Autodesk Inventor part; units mm, degrees
ref_plane "YZ Plane" through (0, 0, 0) normal (1, 0, 0) x (0, 1, 0)
ref_plane "XZ Plane" through (0, 0, 0) normal (0, 1, 0) x (-1, 0, 0)
ref_plane "XY Plane" through (0, 0, 0) normal (0, 0, 1) x (1, 0, 0)
sketch "Boceto1" plane through (0, 0, 0) normal (0, 1, 0) x (-1, 0, 0)
  line L0 (100, 80) -> (-100, 80)
  line L1 (-100, 80) -> (-100, -80)
  line L2 (-100, -80) -> (100, -80)
  line L3 (100, -80) -> (100, 80)
  line L4 (100, 80) -> (-100, -80) construction
  line L5 (-100, 80) -> (100, -80) construction
  point P0 (0, 0)
  dimension "d0" = 200
  dimension "d1" = 160
extrude "Extrusión1" add sketch "Boceto1" along normal blind 20
sketch "Boceto2" plane through (0, 20, 0) normal (0, 1, 0) x (1, 0, 0)
  circle A0 centre (-90, -57.83) radius 3.5
  line L0 (-100, -65.43) -> (-32, -65.43)
  line L1 (-32, -65.43) -> (-32, 14.57)
  line L2 (-32, 14.57) -> (-100, 14.57)
  line L3 (-100, 14.57) -> (-100, -65.43)
  line L4 (-66, -65.43) -> (-66, -8.508)
  circle A1 centre (-66, -57.83) radius 3.5
  circle A2 centre (-42, -57.83) radius 3.5
  line L5 (-32, -25.43) -> (-48.2072, -25.43)
  circle A3 centre (-42, 6.97) radius 3.5
  circle A4 centre (-66, 6.97) radius 3.5
  circle A5 centre (-90, 6.97) radius 3.5
  circle A6 centre (-60, 55) radius 5
  line L6 (-100, 80) -> (-100, -80)
  line L7 (0, 0) -> (0, -20.5185)
  circle A7 centre (90, -57.83) radius 3.5
  circle A8 centre (66, -57.83) radius 3.5
  circle A9 centre (42, -57.83) radius 3.5
  line L8 (100, -65.43) -> (32, -65.43)
  line L9 (66, -65.43) -> (66, -8.508)
  line L10 (32, -25.43) -> (48.2072, -25.43)
  circle A10 centre (90, 6.97) radius 3.5
  line L11 (100, 14.57) -> (100, -65.43)
  circle A11 centre (66, 6.97) radius 3.5
  line L12 (32, 14.57) -> (100, 14.57)
  line L13 (32, -65.43) -> (32, 14.57)
  circle A12 centre (42, 6.97) radius 3.5
  circle A13 centre (60, 55) radius 5
  line L14 (100, 80) -> (100, -80)
  dimension "d4" = 7
  dimension "d5" = 68
  dimension "d6" = 80
  dimension "d7" = 7.6
  dimension "d8" = 10
  dimension "d9" = 7
  dimension "d10" = 24
  dimension "d11" = 10
  dimension "d16" = 0
  dimension "d19" = 40
extrude "Extrusión2" cut sketch "Boceto2" against normal blind 20 contours A0 | A1 L4 | L4 A1 | A2 | A3 | A4 | A5 | A7 | A8 L9 | L9 A8 | A9 | A10 | A11 | A12
sketch "Boceto3" plane through (-100, 0, 80) normal (0, 0, 1) x (1, 0, 0)
  line L0 (0, 20) -> (30, 20)
  line L1 (30, 20) -> (30, 10)
  line L2 (30, 10) -> (0, 10)
  line L3 (0, 10) -> (0, 20)
  line L4 (100, 0) -> (100, 11.6249)
  line L5 (200, 20) -> (170, 20)
  line L6 (170, 20) -> (170, 10)
  line L7 (170, 10) -> (200, 10)
  line L8 (200, 10) -> (200, 20)
  dimension "d22" = 30
  dimension "d23" = 10
extrude "Extrusión3" add sketch "Boceto3" along normal blind 40
sketch "Boceto4" plane through (0, 20, 0) normal (0, 1, 0) x (1, 0, 0)
  line L0 (-60, 60) -> (-60, 50)
  line L1 (-70, 50) -> (-70, 60)
  line L2 (-60, 50) -> (-70, 60) construction
  line L3 (-70, 50) -> (-60, 60) construction
  line L4 (-60, 50) -> (-70, 50)
  circle A0 centre (-68.25, 51.75) radius 1.75
  line L5 (-70, 60) -> (-60, 60)
  circle A1 centre (-61.75, 58.25) radius 1.75
  line L6 (100, 80) -> (-100, 80)
  line L7 (0, 80) -> (0, 60)
  line L8 (60, 60) -> (60, 50)
  circle A2 centre (61.75, 58.25) radius 1.75
  line L9 (70, 60) -> (60, 60)
  line L10 (70, 50) -> (70, 60)
  line L11 (60, 50) -> (70, 60) construction
  line L12 (70, 50) -> (60, 60) construction
  line L13 (60, 50) -> (70, 50)
  circle A3 centre (68.25, 51.75) radius 1.75
  line L14 (-100, 80) -> (-100, -120)
  line L15 (100, 80) -> (100, -120)
  point P0 (0, 0)
  point P1 (-70.0286, 64.971)
  point P2 (-65, 50)
  point P3 (70.0286, 64.971)
  point P4 (65, 50)
  dimension "d26" = 1.75
  dimension "d27" = 8.25
  dimension "d28" = 20
  dimension "d29" = 10
  dimension "d30" = 10
  dimension "d31" = 1.75
  dimension "d32" = 1.75
  dimension "d33" = 1.75
  dimension "d58" = 30
  dimension "d59" = 30
extrude "Extrusión4" cut sketch "Boceto4" against normal blind 40 contours A1 | A0 | A2 | A3
sketch "Boceto5" plane through (0, 20, 0) normal (0, 1, 0) x (1, 0, 0)
  line L0 (-100, -80) -> (-100, -120)
  line L1 (-70.0001, -120) -> (-70.0001, -80)
  line L2 (-55.1959, -79.9497) -> (-70.0001, -80)
  line L3 (-70.0001, -80) -> (-100, -80)
  line L4 (-100, -120) -> (-70.0001, -120)
  line L5 (-64.3507, -80) -> (-74.3507, -80)
  circle A0 centre (-81.75, -108.25) radius 1.75
  circle A1 centre (-88.25, -101.75) radius 1.75
  line L6 (-70.0001, -80) -> (70.0001, -80)
  line L7 (0, -80) -> (0, -101.75)
  circle A2 centre (81.75, -108.25) radius 1.75
  circle A3 centre (88.25, -101.75) radius 1.75
  line L8 (-70, -80) -> (70, -80)
  line L9 (-100, 80) -> (-100, -120)
  point P0 (0, 0)
  point P1 (-81.75, -101.75)
  point P2 (-63.4459, -118.25)
  point P3 (81.75, -101.75)
  dimension "d36" = 11.7499
  dimension "d37" = 40
  dimension "d38" = 29.9999
  dimension "d39" = 21.75
  dimension "d40" = 11.75
  dimension "d41" = 28.3003
  dimension "d42" = 11.7499
  dimension "d43" = 0
  dimension "d44" = 0
hole "Agujero1" at (-88.25, 20, 101.75) at (-81.75, 20, 108.25) at (81.75, 20, 108.25) at (88.25, 20, 101.75) direction (0, -1, 0) diameter 3.5 end through all
ref_plane "Plano de trabajo1" through (100, 0, 0) normal (0, 0, -1) x (-1, 0, 0)
ref_plane "Plano de trabajo2" through (0, 0, -80) normal (-1, 0, 0) x (0, 0, 1)
sketch "Boceto6" plane through (0, 0, 0) normal (0, -1, 0) x (1, 0, 0)
  circle A0 centre (10, -10) radius 1.75
  line L0 (6.803, 0) -> (14.6069, 0)
  line L1 (0, 0) -> (0, -4.8284)
  line L2 (0, 0) -> (20.0354, 0)
  circle A1 centre (10, 10) radius 1.75
  line L3 (0, 0) -> (0, 4.8284)
  circle A2 centre (-10, 10) radius 1.75
  circle A3 centre (-10, -10) radius 1.75
  dimension "d63" = 3.5
  dimension "d64" = 10
  dimension "d65" = 10
hole "Agujero2" at (10, 0, 10) at (-10, 0, 10) at (-10, 0, -10) at (10, 0, -10) direction (0, 1, 0) diameter 3.5 end through all
sketch "Boceto7" plane through (0, 0, 0) normal (0, -1, 0) x (1, 0, 0)
  line L0 (-16, 16) -> (16, 16)
  line L1 (16, 16) -> (16, -16)
  line L2 (16, -16) -> (-16, -16)
  line L3 (-16, -16) -> (-16, 16)
  line L4 (-16, 16) -> (16, -16) construction
  line L5 (16, 16) -> (-16, -16) construction
  point P0 (0, 0)
  point P1 (0, 0)
  point P2 (0, 0)
  dimension "d73" = 32
  dimension "d74" = 32
extrude "Extrusión5" cut sketch "Boceto7" against normal blind 10
sketch "Boceto8" plane through (0, 20, 0) normal (0, 1, 0) x (1, 0, 0)
  line L0 (-15, -60) -> (15, -60)
  circle A0 centre (10, -65) radius 1.75
  line L1 (-10, -65) -> (10, -65)
  line L2 (15, -60) -> (15, -70)
  circle A1 centre (-10, -65) radius 1.75
  line L3 (-15, -70) -> (15, -60) construction
  line L4 (-15, -60) -> (15, -70) construction
  line L5 (-15, -70) -> (-15, -60)
  line L6 (15, -70) -> (-15, -70)
  point P0 (0, 0)
  point P1 (0, -69.1269)
  point P2 (-15, -67.1661)
  point P3 (0, -69.1269)
  point P4 (15, -65)
  dimension "d77" = 10
  dimension "d78" = 30
  dimension "d79" = 5
  dimension "d80" = 5
  dimension "d81" = 5
  dimension "d82" = 5
hole "Agujero3" at (-10, 20, 65) at (10, 20, 65) direction (0, -1, 0) diameter 3.5 end through all
split "Dividir1" plane through (100, 0, 0) removes the side toward (0, 0, 1)
split "Dividir2" plane through (0, 0, -80) removes the side toward (-1, 0, 0)
properties part number "base_back_2"
Can you work these out from the model? Positions are in its coordinate system, mm. A direction names the side the tool comes from. Give positions to 0.01 mm unless a question says otherwise; leave off trailing zeros. Write each loop counter-clockwise with the first axis right and the second up, starting at its lowest first coordinate (ties: lowest second). Pieces come first, ordered by that corner, then holes. Notation, with made-up numbers: M -35.5,7 L -20.5,7 A24 ccw -20.5,27 Z; hole C 22.25,36.25 d4. An arc over 180 degrees is marked long. Answer in a Markdown table with one row per item. Add a question column.
Item 1: Imagine slicing it at D-D, the plane y = 7.75. Write out the boundary of the cut face in (x, z).
Item 2: On a 3-axis mill with a long thin cutter (end or side, diameter ignored), from which of +Z, -Z, +X, -X, +Y, -Y can I reach the whole of each face in a straight line? I mean faces 5 (the cylindrical face through (8.5, 15.1, -10.9)), 6 (the flat face through (8, 10, -8)). Say none if no direction works.
Item 3: We'd pull the mould along Z, two halves only. Please class faces 1 (the cylindrical face through (38.503, 10.14, -7.124)), 2 (the cylindrical face through (62.503, 10.14, -7.124)), 3 (the flat face through (51, 10, -80)), 4 (the flat face through (8, 5, -16)): released by +Z, released by -Z, zero draft, split by the parting line, or undercut.
Item 4: Please list where these lines run through material, in increasing order: L1, parallel to X at y = 16, z = -6.97; L2, parallel to X at y = 6.5, z = -6.97; L3, parallel to Z at x = 90, y = 2.
Item 5: For pin 1 Ø9 at (x, z) = (42, -6.97) entering from -Y, with a flat end and sliding along its axis, tell me the tip position at first contact or that it passes through.
Item 6: Imagine slicing it at B-B, the plane x = 90. Write out the boundary of the cut face in (y, z).
Item 7: Imagine slicing it at C-C, the plane z = -6.97. Write out the boundary of the cut face in (x, y).
Item 8: Imagine slicing it at A-A, the plane z = -51.75. Write out the boundary of the cut face in (x, y), plus the area to 3 significant figures.
Evaluation:
| question | item | result |
|---|---|---|
| 1 | outline | M 0,-80 L 100,-80 L 100,0 L 16,0 L 16,-16 L 0,-16 Z; hole C 42,-6.97 d7; hole C 61.75,-58.25 d3.5; hole C 66,-6.97 d7; hole C 68.25,-51.75 d3.5; hole C 90,-6.97 d7 |
| 2 | face 5 | +Y, -Y |
| 2 | face 6 | +Z, -X, -Y |
| 3 | face 1 | undercut |
| 3 | face 2 | undercut |
| 3 | face 3 | released by -Z |
| 3 | face 4 | released by +Z |
| 4 | L1 | x = 0 to 38.5, 45.5 to 62.5, 69.5 to 86.5, 93.5 to 100 |
| 4 | L2 | x = 16 to 38.5, 45.5 to 62.5, 69.5 to 86.5, 93.5 to 100 |
| 4 | L3 | z = -80 to -10.47, -3.47 to 0 |
| 5 | pin 1 | stops at y = 0 |
| 6 | outline | M 0,-80 L 20,-80 L 20,-10.47 L 0,-10.47 Z; M 0,-3.47 L 20,-3.47 L 20,0 L 0,0 Z |
| 7 | outline | M 0,10 L 16,10 L 16,0 L 38.5,0 L 38.5,20 L 0,20 Z; M 45.5,0 L 62.5,0 L 62.5,20 L 45.5,20 Z; M 69.5,0 L 86.5,0 L 86.5,20 L 69.5,20 Z; M 93.5,0 L 100,0 L 100,20 L 93.5,20 Z |
| 8 | outline | M 0,0 L 66.5,0 L 66.5,20 L 0,20 Z; M 70,0 L 100,0 L 100,20 L 70,20 Z |
| 8 | area | 1,930 mm² |
